The listing builds one solid part. Answer for the finished solid, in the listing's coordinates (mm). A direction names the side the tool comes from. Coordinates: 2 decimals unless noted, no trailing zeros. Order: outer loops, then holes, each group sorted by start corner. A loop starts at its lowest first (then second) coordinate and runs counter-clockwise, first axis right, second up. Notation, with made-up numbers: (45.25, 69) -> (101.25, 69) arc R28 ccw to (101.25, 103) -> close; hole circle Ø10 at (69.5, 56.5). An arc over 180 degrees is marked (long way). Return JSON: item names as keys, results as strings.
from build123d import *

# Parameters (mm, degrees)
ESQUISSE1_R                                   = 5
BOSS_EXTRU_1_DEPTH                            = 40
ESQUISSE2_R                                   = 3
BOSS_EXTRU_2_DEPTH                            = 10
TROU_POUR_TARAUDAGE_POUR_TROU_TARAUD_M5_D     = 4.2
TROU_POUR_TARAUDAGE_POUR_TROU_TARAUD_M5_DEPTH = 10
TROU_POUR_TARAUDAGE_POUR_TROU_TARAUD_M5_TIP   = 1.2618073
CHANFREIN1_SIZE                               = 0.5


with BuildPart() as part:
    # Esquisse1 → Boss.-Extru.1 (new body)
    with BuildSketch(Plane.XY):
        Circle(ESQUISSE1_R)
    extrude(amount=BOSS_EXTRU_1_DEPTH)

    # Esquisse2 → Boss.-Extru.2 (add)
    with BuildSketch(Plane(origin=(0, 0, 0), x_dir=(-1, 0, 0), z_dir=(0, 0, -1))):
        Circle(ESQUISSE2_R)
    extrude(amount=BOSS_EXTRU_2_DEPTH)

    # Trou pour taraudage pour trou taraudé M51
    with Locations(Plane.XY.offset(40)):
        with Locations((0, 0)):
            Hole(TROU_POUR_TARAUDAGE_POUR_TROU_TARAUD_M5_D / 2, depth=TROU_POUR_TARAUDAGE_POUR_TROU_TARAUD_M5_DEPTH)
            with Locations((0, 0, -(TROU_POUR_TARAUDAGE_POUR_TROU_TARAUD_M5_DEPTH + TROU_POUR_TARAUDAGE_POUR_TROU_TARAUD_M5_TIP / 2))):  # 118° drill point
                Cone(0, TROU_POUR_TARAUDAGE_POUR_TROU_TARAUD_M5_D / 2, TROU_POUR_TARAUDAGE_POUR_TROU_TARAUD_M5_TIP, mode=Mode.SUBTRACT)

    # Chanfrein1
    chanfrein1_edges = [part.edges().sort_by_distance(p)[0] for p in [
        (-5, 0, 0),
        (-5, 0, 40),
        (3, 0, -10),
    ]]
    chamfer(chanfrein1_edges, length=CHANFREIN1_SIZE)


solid = part.part
1. Consider line 1 (Y direction, x = 0, z = 33.5); line 2 (Z direction, x = 1.75, y = -4); line 3 (Y direction, x = 0.25, z = 22). Determine where each line is inside the solid, lowest interval first. Write a range as from..to.
Answer block:
{"line 1": "y = -5..-2.1, 2.1..5", "line 2": "z = 0..40", "line 3": "y = -4.99..4.99"}
2. Determine the mould class of faces 4 (the face through (-1.08, -4.88, 19.73)), 5 (the face through (1, -3, 0)), 6 (the face through (0.35, 0.11, 28.96)) for opening direction Y: pulls with the +Y half, pulls with the -Y half, needs draft (parallel to the pull), parting line crosses it, or undercut.
Answer block:
{"face 4": "parting line crosses it", "face 5": "needs draft", "face 6": "undercut"}
3. For faces 1 (the face through (3, 0, -5)), 2 (the face through (-2.003, 0.631, 34.93)), 3 (the face through (0, 0, -10)), determine the directions among +Z, -Z, +X, -X, +Y, -Y from which every point of the face is accessible in a straight line to the end or side of a thin tool.
Answer block:
{"face 1": "-Z", "face 2": "+Z", "face 3": "-Z, +X, -X, +Y, -Y"}
4. The part is cut by section A-A on z = -5. Give the vertices of the cut face in (x, y).
Answer block:
{"outline": "circle Ø6 at (0, 0)"}
5. Each of these flat-tipped pins is pushed along its axis until it touches: pin 1 Ø1 at (x, z) = (-3.5, 4.5) entering from +Y; pin 2 Ø4 at (x, z) = (4, -4.5) entering from -Y; pin 3 Ø3 at (x, z) = (-2, -1) entering from +Y. Where does it stop, or does it pass through?
Answer block:
{"pin 1": "stops at y = 4", "pin 2": "stops at y = -2.24", "pin 3": "stops at y = 4.68"}
6. The part is cut by section B-B on z = 24. Give the vertices of the cut face in (x, y).
Answer block:
{"outline": "circle Ø10 at (0, 0)"}
